Can you work these out from the drawing? Everything is in mm from the part's minimum corner. A direction names the side the tool comes from. Round coordinates to 2 decimals unless told otherwise and drop trailing zeros. Write each loop counter-clockwise with the first axis right and the second up, starting at its lowest first coordinate (ties: lowest second). Pieces come first, ordered by that corner, then holes.
Q1. Please list where these lines run through material, in increasing order: line 1 along Z through (x, y) = (45.5, 222.5); line 2 along Y through (x, z) = (30, 54); line 3 along Z through (x, y) = (45, 80.5).
Q2. I'm going to push flat-ended pins straight in: pin 1 Ø2 at (x, z) = (71, 134) entering from -Y; pin 2 Ø1 at (x, z) = (47.5, 163.5) entering from -Y; pin 3 Ø1 at (x, y) = (70, 135) entering from +Z. Where does each tip first touch, or does it pass through?
Q3. If we section it at B-B (y = 40): Please give me the cut outline in (x, z).
Q4. If we section it at A-A (x = 45): Please give me the cut outline in (y, z), plus the area to 3 significant figures.
Q5. If we section it at C-C (z = 172): Please give me the cut outline in (x, y), plus the area to 3 significant figures.
Q6. For the marked faces 1 and 2, which set-ups out of +Z, -Z, +X, -X, +Y, -Y let a thin tool reach every point of the face, with its end or its side?
Q7. If we section it at D-D (x = 26.5): Please give me the cut outline in (y, z), plus the area to 3 significant figures.
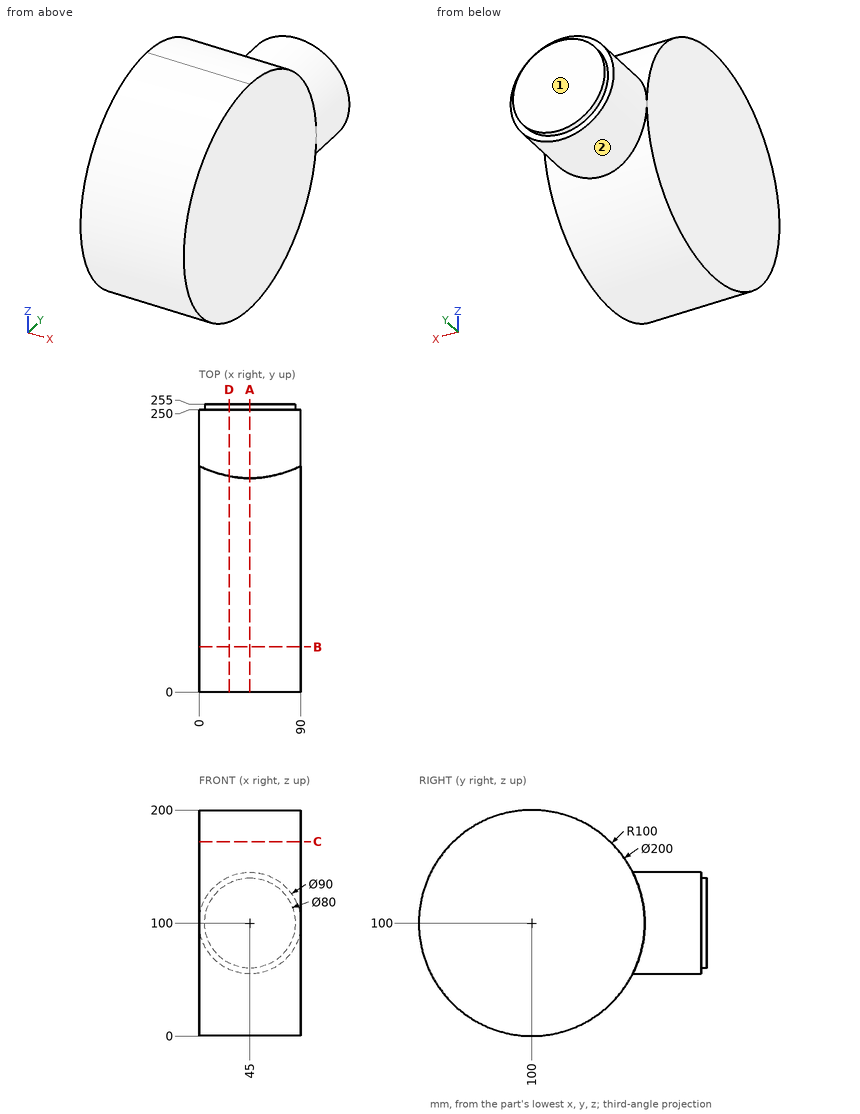
A:
1. line 1: z = 55 to 145
1. line 2: y = 11.21 to 188.79
1. line 3: z = 1.92 to 198.08
2. pin 1: stops at y = 5.6
2. pin 2: stops at y = 22.34
2. pin 3: stops at z = 193.86
3. outline: (0, 20) - (90, 20) - (90, 180) - (0, 180) - close
4. outline: (189.3, 55) - (250, 55) - (250, 60) - (255, 60) - (255, 140) - (250, 140) - (250, 145) - (189.3, 145) arc R100 ccw (long way) to start
4. area: 36,600 mm2
5. outline: (0, 30.6) - (90, 30.6) - (90, 169.4) - (0, 169.4) - close
5. area: 12,500 mm2
6. face 1: +Z, -Z, +X, -X, +Y
6. face 2: +Y
7. outline: (191.2, 58.98) - (250, 58.98) - (250, 64.54) - (255, 64.54) - (255, 135.46) - (250, 135.46) - (250, 141.02) - (191.2, 141.02) arc R100 ccw (long way) to start
7. area: 36,100 mm2
